Source: CAD feature listing. Evaluate the final solid. Frame: model axes, mm. Coordinates: 2 decimals unless noted, no trailing zeros. Order: outer loops, then holes, each group sorted by start corner. A loop starts at its lowest first (then second) coordinate and runs counter-clockwise, first axis right, second up. Notation, with made-up numbers: (70, 59) - (78, 59) arc R21 cw to (78, 94) - close; hole circle Ø4 at (-27, 2). An arc over 180 degrees is marked (long way). One line per question, with ' | ' between items. Start each with the question number.
(1) Line query: line 1 along Y through (x, z) = (6.35, 0.65) (3 decimals); line 2 along Y through (x, z) = (19.75, 1) (3 decimals). Output: solid intervals per line, ascending.
(2) Section B-B (z = 1.75). Return the cut outline in (x, y) (3 decimals).
(3) Section A-A (x = 19.05). Return the cut outline in (y, z) (3 decimals).
(4) Draft query along Y for faces 1 (the flat face through (13, -3.175, 2)), 2 (the cylindrical face through (17.78, 3.23, 1.61)), 3 (the flat face through (13, 5, 3.175)), 4 (the flat face through (13, 12.7, 2)). Return one class per face: +Y half, -Y half, draft (parallel to the pull), parting line (faces both ways), or undercut.
from build123d import *

# Parameters (mm, degrees)
BOSS_EXTRUDE1_DEPTH = 25.4
SKETCH2_R           = 1.27
CUT_EXTRUDE1_DEPTH  = 25.4
SKETCH3_W           = 25.4
SKETCH3_H           = 3.175
CUT_EXTRUDE2_DEPTH  = 10.668


with BuildPart() as part:
    # Sketch1 → Boss-Extrude1 (new body)
    with BuildSketch(Plane(origin=(0, 0, 0), x_dir=(0, 0, -1), z_dir=(1, 0, 0))):
        Polygon((0, 0), (0, 12.7), (-3.175, 12.7), (-3.175, -3.175), (10.668, -3.175), (10.668, 0), align=None)
    extrude(amount=BOSS_EXTRUDE1_DEPTH)

    # Sketch2 → Cut-Extrude1 (cut)
    with BuildSketch(Plane.XY.offset(3.175)):
        with Locations((6.35, 3.175)):
            Circle(SKETCH2_R)
        with Locations((19.05, 3.175)):
            Circle(SKETCH2_R)
    extrude(amount=-CUT_EXTRUDE1_DEPTH, mode=Mode.SUBTRACT)

    # Sketch3 → Cut-Extrude2 (cut)
    with BuildSketch(Plane(origin=(0, 0, -10.668), x_dir=(-1, 0, 0), z_dir=(0, 0, -1))):
        with Locations((-12.7, -1.5875)):
            Rectangle(SKETCH3_W, SKETCH3_H)
    extrude(amount=-CUT_EXTRUDE2_DEPTH, mode=Mode.SUBTRACT)


solid = part.part
Response values:
1) line 1: y = -3.175 to 1.905, 4.445 to 12.7 | line 2: y = -3.175 to 2.115, 4.235 to 12.7
2) outline: (0, -3.175) - (25.4, -3.175) - (25.4, 12.7) - (0, 12.7) - close; hole circle Ø2.54 at (6.35, 3.175); hole circle Ø2.54 at (19.05, 3.175)
3) outline: (-3.175, 0) - (1.905, 0) - (1.905, 3.175) - (-3.175, 3.175) - close; (4.445, 0) - (12.7, 0) - (12.7, 3.175) - (4.445, 3.175) - close
4) face 1: -Y half | face 2: undercut | face 3: draft | face 4: +Y half
